Work out the finished part from the listing and answer in its coordinate system (mm). A direction names the side the tool comes from. Coordinates: 2 decimals unless noted, no trailing zeros. Loops run counter-clockwise (first coordinate to the right, second up) from the corner with the lowest first, then second, coordinate; pieces in that order, holes last. Notation, with made-up numbers: (-38, -34.75) -> (5, -34.75) arc R18 cw to (5, -22.75) -> close; hole circle Ø9 at (60.5, 40.25). An arc over 180 degrees is marked (long way). Use a Markdown table: item, result. Add a question column.
```python
from build123d import *

# Parameters (mm, degrees)
DOME1_FACE_RADIUS          = 3
DOME1_HEIGHT               = 1
MIRROR1_COPY_1_FACE_RADIUS = 3
MIRROR1_COPY_1_HEIGHT      = 1
FILLET1_R                  = 0.25


with BuildPart() as part:
    # Sketch1 → Revolve1 (revolve)
    with BuildSketch(Plane.XY, mode=Mode.PRIVATE) as revolve1_sk:
        Polygon((0, 0), (0, 5.5), (-3, 5.5), (-3, 5), (-2.5, 5), (-2.5, 0), align=None)
    revolve1 = revolve(revolve1_sk.sketch.rotate(Axis((0, 0, 0), (0, 1, 0)), 270), axis=Axis((0, 0, 0), (0, 1, 0)))

    # Dome1: a dome of height H over a round flat face of radius A is a cap of a sphere of radius (A * A + H * H) / (2 * H)
    dome1_r = (DOME1_FACE_RADIUS * DOME1_FACE_RADIUS + DOME1_HEIGHT * DOME1_HEIGHT) / (2 * DOME1_HEIGHT)
    dome1_base = Plane((0, 5.5, 0), z_dir=(0, 1, 0))
    with Locations(dome1_base.offset(DOME1_HEIGHT - dome1_r)):
        dome1_ball = Sphere(dome1_r, mode=Mode.PRIVATE)
    add(split(dome1_ball, bisect_by=dome1_base, keep=Keep.TOP, mode=Mode.PRIVATE))

    # Mirror1: Revolve1 across plane
    add(revolve1.mirror(Plane(origin=(-2.5, 0, 0), x_dir=(0, 0, 1), z_dir=(0, 1, 0))))

    # Mirror1 copy 1: a dome of height H over a round flat face of radius A is a cap of a sphere of radius (A * A + H * H) / (2 * H)
    mirror1_copy_1_r = (MIRROR1_COPY_1_FACE_RADIUS * MIRROR1_COPY_1_FACE_RADIUS + MIRROR1_COPY_1_HEIGHT * MIRROR1_COPY_1_HEIGHT) / (2 * MIRROR1_COPY_1_HEIGHT)
    mirror1_copy_1_base = Plane((0, -5.5, 0), z_dir=(0, -1, 0))
    with Locations(mirror1_copy_1_base.offset(MIRROR1_COPY_1_HEIGHT - mirror1_copy_1_r)):
        mirror1_copy_1_ball = Sphere(mirror1_copy_1_r, mode=Mode.PRIVATE)
    add(split(mirror1_copy_1_ball, bisect_by=mirror1_copy_1_base, keep=Keep.TOP, mode=Mode.PRIVATE))

    # Fillet1
    fillet1_edges = [part.edges().sort_by_distance(p)[0] for p in [
        (0, -5.5, 3),
        (3, 5.5, 0),
    ]]
    fillet(fillet1_edges, radius=FILLET1_R)


solid = part.part
```
Item 1: Section A-A (y = 2.25) is taken. Determine the outline of the cut face in (x, z).
Item 2: For faces 1 (the face through (-2, -5, 2)), 2 (the face through (-2.974, 5.184, 0.391)), determine the directions among +Z, -Z, +X, -X, +Y, -Y from which every point of the face is accessible in a straight line to the end or side of a thin tool.
Item 3: Find the intervals of material crossed by probe 1 along Y at (x, z) = (1.5, 2.5); probe 2 along Y at (x, z) = (1.75, -2); probe 3 along Z at (x, y) = (-1.75, -2.5), in increasing order.
Item 4: Given pin 1 (1 mm diameter, centred on y = 0.5, z = 2, fed in from -X); pin 2 (2 mm diameter, centred on x = 0.5, y = 3, fed in from -Z); pin 3 (1.5 mm diameter, centred on x = -0.5, z = -2, fed in from -Y), each flat-ended and moving along its own axis, determine where each tip first touches the part or whether it passes through.
Output:
| question | item | result |
|---|---|---|
| 1 | outline | circle Ø5 at (0, 0) |
| 2 | face 1 | none |
| 2 | face 2 | +Y, -Y |
| 3 | probe 1 | y = -5.56 to -5, 5 to 5.56 |
| 3 | probe 2 | y = -5.74 to -5, 5 to 5.74 |
| 3 | probe 3 | z = -1.79 to 1.79 |
| 4 | pin 1 | stops at x = -2 |
| 4 | pin 2 | stops at z = -2.5 |
| 4 | pin 3 | stops at y = -6.32 |
